Autodesk Inventor part; units mm, degrees
ref_plane "YZ Plane" through (0, 0, 0) normal (1, 0, 0) x (0, 1, 0)
ref_plane "XZ Plane" through (0, 0, 0) normal (0, 1, 0) x (-1, 0, 0)
ref_plane "XY Plane" through (0, 0, 0) normal (0, 0, 1) x (1, 0, 0)
sketch "Sketch1" plane through (0, 0, 0) normal (0, 1, 0) x (-1, 0, 0)
  line L0 (-50, -25) -> (50, -25)
  line L1 (50, -25) -> (50, 25)
  line L2 (50, 25) -> (-50, 25)
  line L3 (-50, 25) -> (-50, -25)
  line L4 (-50, -25) -> (50, 25) construction
  line L5 (50, -25) -> (-50, 25) construction
  point P0 (0, 0)
  dimension "d0" = 100
  dimension "d1" = 50
extrude "Extrusion1" add sketch "Sketch1" along normal blind 10
sketch "Sketch2" plane through (0, 0, 0) normal (0, 0, 1) x (1, 0, 0)
  line L0 (-50, 10) -> (50, 10)
  line L1 (31.5957, 10) -> (-31.5209, 10)
  line L2 (15, 10) -> (-15, 10)
  line L3 (-15, 10) -> (-15, 36)
  line L4 (-15, 36) -> (15, 36)
  line L5 (15, 36) -> (15, 10)
  line L6 (15, 10) -> (-15, 36) construction
  line L7 (-15, 10) -> (15, 36) construction
  line L8 (34, 30) -> (-34, 30)
  line L9 (-34, 30) -> (-34, 10)
  line L10 (-34, 10) -> (34, 10)
  line L11 (34, 10) -> (34, 30)
  line L12 (34, 30) -> (-34, 10) construction
  line L13 (-34, 30) -> (34, 10) construction
  line L14 (40, 36) -> (-40, 36)
  line L15 (-40, 36) -> (-40, 10)
  line L16 (-40, 10) -> (40, 10)
  line L17 (40, 10) -> (40, 36)
  line L18 (40, 36) -> (-40, 10) construction
  line L19 (-40, 36) -> (40, 10) construction
  line L20 (-50, 0) -> (50, 0)
  point P0 (0, 0)
  point P1 (0, 23)
  point P2 (0, 20)
  point P3 (0, 23)
  point P4 (-34, 20)
  point P5 (0, 0)
  point P6 (0, 0)
  point P7 (0, 0)
  point P8 (0, 10)
  point P9 (40, 10)
  point P10 (15, 36)
  point P11 (15, 30)
  point P12 (34, 10)
  point P13 (-34, 10)
  point P14 (-15, 30)
  point P15 (-15, 36)
  dimension "d5" = 80
  dimension "d7" = 0
  dimension "d8" = 6
  dimension "d9" = 30
  dimension "d10" = 20
  dimension "d13" = 68
extrude "Extrusion2" add sketch "Sketch2" along normal mid plane 30 contours L15 L14 L3 L8 L9 L0 | L14 L17 L0 L11 L8 L5
properties part number "holder sensor"
Design review of the part built by this model. Coordinates are the model's own, in mm. A direction names the side the tool comes from. Give positions to 0.01 mm unless a question says otherwise; leave off trailing zeros. Loops run counter-clockwise (first coordinate to the right, second up) from the corner with the lowest first, then second, coordinate; pieces in that order, holes last. Notation, with made-up numbers: (49.25, 52.25) - (78.25, 52.25) arc R31 cw to (78.25, 77.25) - close; hole circle Ø4 at (-6.75, -1). An arc over 180 degrees is marked (long way). Use CSV: the item, a comma, the result in double quotes. Start each with the question number.
1. Add section C-C (z = 6.5). State the section outline as (x, y) points.
2. Machinability: for faces 1 (the flat face through (-15, 33, 0)), 2 (the flat face through (36, 29, 15)), 3 (the flat face through (40, 23, 0)), 4 (the flat face through (-36, 29, -15)), which of the approach directions +Z, -Z, +X, -X, +Y, -Y give a long, thin tool a straight path to every point of the face, cutting with its end or side? Answer none if there is none.
3. Add section A-A (x = 25.5). State the section outline as (y, z) points.
4. Add section B-B (y = 14.5). State the section outline as (x, z) points, plus the area to 3 significant figures.
5. Add section D-D (x = -35.5). State the section outline as (y, z) points.
6. Draft analysis for pull direction Y (two halves, no side actions). For faces 5 (the flat face through (1, 10, 0)), 6 (the flat face through (28, 36, 0)), 7 (the flat face through (36, 29, -15)), 8 (the flat face through (25, 30, 0)), state which applies: released by +Y, released by -Y, zero draft, split by the parting line, or undercut.
7. Wall thickness on L1, parallel to Y at x = 28.5, z = 2; L2, parallel to X at y = 15, z = -2; L3, parallel to Y at x = 13, z = 9.5: over which ranges is each line inside the solid? List them lowest first.
8. Insertion check: P1, Ø10, axis at y = 25, z = -0.5, coming from the -X side; P2, Ø25, axis at x = 6, z = -2.5, coming from the +Y side; P3, Ø3, axis at y = 34.5, z = -3.5, coming from the +X side; P4, Ø6, axis at x = -16.5, y = 30, coming from the +Z side. Each pin has a flat end and moves straight along its axis. Give the tip position at first contact, or say it passes through.
Results found:
1,outline,"(-50, 0) - (50, 0) - (50, 10) - (40, 10) - (40, 36) - (15, 36) - (15, 30) - (34, 30) - (34, 10) - (-34, 10) - (-34, 30) - (-15, 30) - (-15, 36) - (-40, 36) - (-40, 10) - (-50, 10) - close"
2,face 1,"+Z, -Z, +Y"
2,face 2,"+Z, +X, -X, +Y"
2,face 3,"+Z, -Z, +X, +Y"
2,face 4,"-Z, +X, -X, +Y"
3,outline,"(0, -25) - (10, -25) - (10, 25) - (0, 25) - close; (30, -15) - (36, -15) - (36, 15) - (30, 15) - close"
4,outline,"(-40, -15) - (-34, -15) - (-34, 15) - (-40, 15) - close; (34, -15) - (40, -15) - (40, 15) - (34, 15) - close"
4,area,"360 mm²"
5,outline,"(0, -25) - (10, -25) - (10, -15) - (36, -15) - (36, 15) - (10, 15) - (10, 25) - (0, 25) - close"
6,face 5,"undercut"
6,face 6,"released by +Y"
6,face 7,"zero draft"
6,face 8,"undercut"
7,L1,"y = 0 to 10, 30 to 36"
7,L2,"x = -40 to -34, 34 to 40"
7,L3,"y = 0 to 10"
8,P1,"stops at x = -40"
8,P2,"stops at y = 36"
8,P3,"stops at x = 40"
8,P4,"stops at z = 15"
